from build123d import *

# Parameters (mm, degrees)
CROQUIS1_W                = 42
CROQUIS1_H                = 42
SALIENTE_EXTRUIR1_DEPTH   = 48
CROQUIS2_R                = 11
CROQUIS2_R_2              = 4.5
SALIENTE_EXTRUIR2_DEPTH   = 3
SALIENTE_EXTRUIR3_DEPTH   = 25
TALADRO_ROSCADO_M31_D     = 2.5
TALADRO_ROSCADO_M31_DEPTH = 8.5
TALADRO_ROSCADO_M31_TIP   = 0.751075774
CHAFL_N1_SIZE             = 4


with BuildPart() as part:
    # Croquis1 → Saliente-Extruir1 (new body)
    with BuildSketch(Plane(origin=(0, 0, 0), x_dir=(1, 0, 0), z_dir=(0, 1, 0))):
        Rectangle(CROQUIS1_W, CROQUIS1_H)
    extrude(amount=SALIENTE_EXTRUIR1_DEPTH)

    # Croquis2 → Saliente-Extruir2 (add)
    with BuildSketch(Plane(origin=(0, 48, 0), x_dir=(1, 0, 0), z_dir=(0, 1, 0))):
        with Locations(Location((0, 0, 0), (0, 0, 270))):
            Circle(CROQUIS2_R)
        with Locations(Location((0, 0, 0), (0, 0, 270))):
            Circle(CROQUIS2_R_2, mode=Mode.SUBTRACT)
    extrude(amount=SALIENTE_EXTRUIR2_DEPTH)

    # Croquis3 → Saliente-Extruir3 (add)
    with BuildSketch(Plane(origin=(0, 48, 0), x_dir=(1, 0, 0), z_dir=(0, 1, 0))):
        with BuildLine():
            Line((1.5, 2), (-1.5, 2))
            ThreePointArc((-1.5, 2), (0, -2.5), (1.5, 2))
        make_face()
    extrude(amount=SALIENTE_EXTRUIR3_DEPTH)

    # Taladro roscado M31
    with Locations(Plane(origin=(0, 48, 0), x_dir=(1, 0, 0), z_dir=(0, 1, 0))):
        with Locations((-15.5, 15.5), (-15.5, -15.5), (15.5, -15.5), (15.5, 15.5)):
            Hole(TALADRO_ROSCADO_M31_D / 2, depth=TALADRO_ROSCADO_M31_DEPTH)
            with Locations((0, 0, -(TALADRO_ROSCADO_M31_DEPTH + TALADRO_ROSCADO_M31_TIP / 2))):  # 118° drill point
                Cone(0, TALADRO_ROSCADO_M31_D / 2, TALADRO_ROSCADO_M31_TIP, mode=Mode.SUBTRACT)

    # Chaflán1
    chafl_n1_edges = [part.edges().sort_by_distance(p)[0] for p in [
        (-21, 24, -21),
        (21, 24, -21),
        (21, 24, 21),
        (-21, 24, 21),
    ]]
    chamfer(chafl_n1_edges, length=CHAFL_N1_SIZE)


solid = part.part
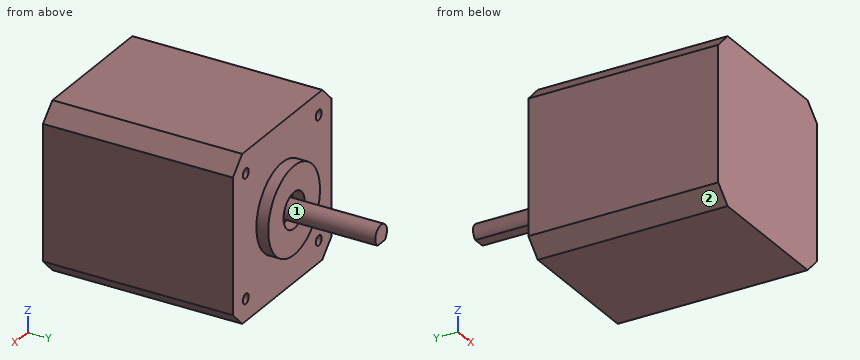
Geometry: final body of the model. Coordinates: model frame, mm. Face numbers are marked on the shaded views. A direction names the side the tool comes from. Coordinates: 2 decimals unless noted, no trailing zeros. Loops run counter-clockwise (first coordinate to the right, second up) from the corner with the lowest first, then second, coordinate; pieces in that order, holes last. Notation, with made-up numbers: M 42.25,31.25 L 71.25,31.25 A27 ccw 71.25,47.25 Z; hole C 38.5,-34 d8. An arc over 180 degrees is marked long. One line per item, written item: value. Start each with the question number.
1) Cut plane C-C (z = 0). Return loops of the section in (x, y), then the cut area to 3 significant figures.
2) Cut plane A-A (y = 49.5). Return loops of the section in (x, z).
3) Pin query (flat end, axial travel): P1, Ø2, axis at x = 3, z = -9, coming from the +Y side; P2, Ø1.5, axis at x = -0.5, y = 57, coming from the -Z side; P3, Ø4, axis at x = 15.5, z = 15.5, coming from the +Y side. Return the tip coordinate at first contact, or that it passes through.
4) Material intervals for L1, parallel to Z at x = -15.5, y = 41; L2, parallel to X at y = 49.9, z = 0, sorted ascending. Write a range as from..to.
5) Cut plane D-D (y = 40.5). Return loops of the section in (x, z), then the cut area to 3 significant figures.
6) Reachability of the marked faces 1 and 2 from +Z, -Z, +X, -X, +Y, -Y: full face, straight path, thin tool, end or side. Return the list, or none.
7) Cut plane B-B (x = 0). Return loops of the section in (y, z).
Evaluation:
1. outline: M -21,0 L 21,0 L 21,48 L 11,48 L 11,51 L 4.5,51 L 4.5,48 L 2.5,48 L 2.5,73 L -2.5,73 L -2.5,48 L -4.5,48 L -4.5,51 L -11,51 L -11,48 L -21,48 Z
1. area: 2,180 mm^2
2. outline: C 0,0 d22; M -1.5,-2 L 1.5,-2 A2.5 ccw long Z; hole C 0,0 d9
3. P1: y = 51
3. P2: z = -2
3. P3: y = 48
4. L1: -21..-16.75, -14.25..14.25, 16.75..21
4. L2: -11..-4.5, -2.5..2.5, 4.5..11
5. outline: M -21,-17 L -17,-21 L 17,-21 L 21,-17 L 21,17 L 17,21 L -17,21 L -21,17 Z; hole C -15.5,-15.5 d2.5; hole C -15.5,15.5 d2.5; hole C 15.5,-15.5 d2.5; hole C 15.5,15.5 d2.5
5. area: 1,710 mm^2
6. face 1: +Y
6. face 2: -Z, -X, +Y, -Y
7. outline: M 0,-21 L 48,-21 L 48,-11 L 51,-11 L 51,-4.5 L 48,-4.5 L 48,-2 L 73,-2 L 73,2.5 L 48,2.5 L 48,4.5 L 51,4.5 L 51,11 L 48,11 L 48,21 L 0,21 Z
